```python
from build123d import *

# Parameters (mm, degrees)
SKETCH1_R               = 34
BOSS_EXTRUDE1_DEPTH     = 7.5
SKETCH4_W               = 44
SKETCH4_H               = 10
BOSS_EXTRUDE2_DEPTH     = 7.5
SKETCH5_R               = 30
SKETCH5_W               = 44
SKETCH5_H               = 2
CUT_EXTRUDE1_DEPTH      = 26.5
SKETCH6_R               = 1.6
CUT_EXTRUDE2_DEPTH      = 30
CUT_EXTRUDE2_DEPTH_BACK = 10


with BuildPart() as part:
    # Sketch1 → Boss-Extrude1 (new body, symmetric)
    with BuildSketch(Plane.XY):
        Circle(SKETCH1_R)
    extrude(amount=BOSS_EXTRUDE1_DEPTH, both=True)

    # Sketch4 → Boss-Extrude2 (add, symmetric)
    with BuildSketch(Plane.XY):
        with Locations((-22, 0)):
            Rectangle(SKETCH4_W, SKETCH4_H)
    extrude(amount=BOSS_EXTRUDE2_DEPTH, both=True)

    # Sketch5 → Cut-Extrude1 (cut)
    with BuildSketch(Plane.XY.offset(7.5)):
        Circle(SKETCH5_R)
        with Locations((-22, 0)):
            Rectangle(SKETCH5_W, SKETCH5_H)
    extrude(amount=-CUT_EXTRUDE1_DEPTH, mode=Mode.SUBTRACT)

    # Sketch6 → Cut-Extrude2 (cut, two sides)
    with BuildSketch(Plane(origin=(0, 5, 0), x_dir=(1, 0, 0), z_dir=(0, 1, 0))) as cut_extrude2_sk:
        with Locations((-40, 0)):
            Circle(SKETCH6_R)
    extrude(amount=CUT_EXTRUDE2_DEPTH, mode=Mode.SUBTRACT)
    extrude(cut_extrude2_sk.sketch, amount=-CUT_EXTRUDE2_DEPTH_BACK, mode=Mode.SUBTRACT)


solid = part.part
```
Could you check a few things on this model? Use its own coordinates, in mm. A direction names the side the tool comes from. Give positions to 0.01 mm unless a question says otherwise; leave off trailing zeros. Write each loop counter-clockwise with the first axis right and the second up, starting at its lowest first coordinate (ties: lowest second). Pieces come first, ordered by that corner, then holes. Notation, with made-up numbers: (35, -9.5) - (60, -9.5) arc R26 cw to (60, 20.5) - close; hole circle Ø9 at (61.5, 82). An arc over 180 degrees is marked (long way). One line per item, written item: value. Start each with the question number.
Item 1: Imagine slicing it at D-D, the plane y = -24. List the corners of the cut face in (x, z) for me, and give its area (3 significant figures).
Item 2: I'm going to push flat-ended pins straight in: pin 1 (5 mm diameter, centred on x = -40, z = 0, fed in from -Y); pin 2 (2 mm diameter, centred on x = 12.5, z = 4.5, fed in from -Y); pin 3 (8 mm diameter, centred on x = 20, y = 12, fed in from +Z) (3 decimals); pin 4 (6 mm diameter, centred on y = -14, z = 2.5, fed in from -X). Where does each tip first touch, or does it pass through?
Item 3: Imagine slicing it at C-C, the plane x = 0. List the corners of the cut face in (y, z) for me, and give its area (3 significant figures).
Item 4: Please list where these lines run through material, in increasing order: line 1 (Z direction, x = -40, y = -2.05); line 2 (X direction, y = 3, z = 0); line 3 (Y direction, x = -36.5, z = -5.75). Write a range as from..to.
Item 5: If we mould it in two halves opening along Z, with no side actions, what happens to faces 1 (the face through (-17, -25, 7.5)), 2 (the face through (-41.18, -2.97, -1.08)), 3 (the face through (-38, -5, 0))? For each: +Z half, -Z half, draft (parallel to the pull), parting line (faces both ways), or undercut.
Item 6: Which directions (+Z, -Z, +X, -X, +Y, -Y) give clear straight access to the entire face, cutting with the end or side of a thin tool? Please do faces 4 (the face through (-44, 3, 0)), 5 (the face through (-38, 5, 0)), 6 (the face through (-37, 1, 0)).
Item 7: Imagine slicing it at A-A, the plane z = 0. List the corners of the cut face in (x, y) for me, and give its area (3 significant figures).
Item 8: Imagine slicing it at B-B, the plane x = -40. List the corners of the cut face in (y, z) for me.
Geometry says:
1. outline: (-24.08, -7.5) - (-18, -7.5) - (-18, 7.5) - (-24.08, 7.5) - close; (18, -7.5) - (24.08, -7.5) - (24.08, 7.5) - (18, 7.5) - close
1. area: 182 mm^2
2. pin 1: y = -5
2. pin 2: y = -32
2. pin 3: through
2. pin 4: x = -32.17
3. outline: (-34, -7.5) - (-30, -7.5) - (-30, 7.5) - (-34, 7.5) - close; (30, -7.5) - (34, -7.5) - (34, 7.5) - (30, 7.5) - close
3. area: 120 mm^2
4. line 1: -7.5..-1.6, 1.6..7.5
4. line 2: -44..-41.6, -38.4..-29.85, 29.85..33.87
4. line 3: -5..-1, 1..5
5. face 1: +Z half
5. face 2: undercut
5. face 3: draft
6. face 4: +Z, -Z, -X, +Y, -Y
6. face 5: +Z, -Z, -X, +Y
6. face 6: +Z, -Z, -X
7. outline: (-44, -5) - (-41.6, -5) - (-41.6, -1) - (-44, -1) - close; (-44, 1) - (-41.6, 1) - (-41.6, 5) - (-44, 5) - close; (-38.4, -5) - (-33.63, -5) arc R34 ccw (long way) to (-33.63, 5) - (-38.4, 5) - (-38.4, 1) - (-29.98, 1) arc R30 cw (long way) to (-29.98, -1) - (-38.4, -1) - close
7. area: 852 mm^2
8. outline: (-5, -7.5) - (-1, -7.5) - (-1, -1.6) - (-5, -1.6) - close; (-5, 1.6) - (-1, 1.6) - (-1, 7.5) - (-5, 7.5) - close; (1, -7.5) - (5, -7.5) - (5, -1.6) - (1, -1.6) - close; (1, 1.6) - (5, 1.6) - (5, 7.5) - (1, 7.5) - close
